from build123d import *

# Parameters (mm, degrees)
MAIN_DEPTH         = 5
SKETCH2_R          = 1.25
FIXHOLE1_DEPTH     = 51
SKETCH3_R          = 1.25
FIXHOLE2_DEPTH     = 51
WINDOWSLOT1_DEPTH  = 2
SKETCH6_R          = 1.25
CUT_EXTRUDE2_DEPTH = 3
LPATTERN1_COUNT    = 5
LPATTERN1_PITCH    = 10
SKETCH7_R          = 1.25
CUT_EXTRUDE3_DEPTH = 11
LPATTERN2_COUNT    = 4
LPATTERN2_PITCH    = 14.142


with BuildPart() as part:
    # Sketch1 → Main (new body, symmetric)
    with BuildSketch(Plane.XY):
        Polygon((-25, -25), (25, 25), (25, 15), (35, 15), (35, 10), (25, 10), (-10, -25), (-10, -35), (-15, -35), (-15, -25), align=None)
    extrude(amount=MAIN_DEPTH, both=True)

    # Sketch2 → FixHole1 (cut, through all)
    with BuildSketch(Plane(origin=(25, 0, 0), x_dir=(0, 0, -1), z_dir=(1, 0, 0))):
        with Locations((0, -30)):
            Circle(SKETCH2_R)
        with Locations((0, 20)):
            Circle(SKETCH2_R)
    extrude(amount=-FIXHOLE1_DEPTH, mode=Mode.SUBTRACT)

    # Sketch3 → FixHole2 (cut, through all)
    with BuildSketch(Plane(origin=(0, -25, 0), x_dir=(-1, 0, 0), z_dir=(0, -1, 0))):
        with Locations((20, 0)):
            Circle(SKETCH3_R)
        with Locations((-30, 0)):
            Circle(SKETCH3_R)
    extrude(amount=-FIXHOLE2_DEPTH, mode=Mode.SUBTRACT)

    # Sketch4 → WindowSlot1 (cut)
    with BuildSketch(Plane.XY.offset(5)):
        Polygon((25, 22.171572875), (-22.171572875, -25), (-18.636038969, -25), (25, 18.636038969), align=None)
    extrude(amount=-WINDOWSLOT1_DEPTH, mode=Mode.SUBTRACT)

    # Sketch6 → Cut-Extrude2 (cut)
    with BuildSketch(Plane(origin=(7.5, -7.5, 0), x_dir=(0, 0, 1), z_dir=(-0.707106781, 0.707106781, 0))):
        with Locations((0, 20)):
            Circle(SKETCH6_R)
    cut_extrude2 = extrude(amount=CUT_EXTRUDE2_DEPTH, mode=Mode.SUBTRACT)

    # LPattern1: Cut-Extrude2 ×5
    with Locations(*[Vector(-0.707106781, -0.707106781, 0) * (i * LPATTERN1_PITCH) for i in range(1, LPATTERN1_COUNT)]):
        add(cut_extrude2, mode=Mode.SUBTRACT)

    # Sketch7 → Cut-Extrude3 (cut, through all)
    with BuildSketch(Plane(origin=(0, 0, -5), x_dir=(-1, 0, 0), z_dir=(0, 0, -1))):
        with Locations((10, -20)):
            Circle(SKETCH7_R)
    cut_extrude3 = extrude(amount=-CUT_EXTRUDE3_DEPTH, mode=Mode.SUBTRACT)

    # LPattern2: Cut-Extrude3 ×4
    with Locations(*[Vector(0.707106781, 0.707106781, 0) * (i * LPATTERN2_PITCH) for i in range(1, LPATTERN2_COUNT)]):
        add(cut_extrude3, mode=Mode.SUBTRACT)


solid = part.part
CAD build for the part. Positions are in the model's coordinates, mm. A direction names the side the tool comes from. Give positions to 0.01 mm unless a question says otherwise; leave off trailing zeros. Write each loop counter-clockwise with the first axis right and the second up, starting at its lowest first coordinate (ties: lowest second). Pieces come first, ordered by that corner, then holes. Notation, with made-up numbers: (-10, -15.5) - (41, -15.5) arc R16 ccw to (41, 13.5) - close; hole circle Ø10 at (16, 26.5). An arc over 180 degrees is marked (long way). Answer as CSV lines item,"result".
Q1. Flat gauge pins, fed straight in: pin 1 Ø2 at (x, z) = (30, 0) entering from +Y; pin 2 Ø10 at (x, y) = (-6.5, 0) entering from -Z; pin 3 Ø2 at (x, z) = (15, -1) entering from -Y; pin 4 Ø2 at (x, z) = (10, 3.5) entering from -Y. Where does each tip first touch, or does it go through?
Result set:
pin 1,"through"
pin 2,"z = -5"
pin 3,"y = -1"
pin 4,"y = -6"
Q2. Pull direction X, two halves, no side cores. Call faces 4 (the face through (35, 13, 0)), 5 (the face through (-12, -35, 0)), 6 (the face through (0.26, -12.65, -0.16)): released by +X, released by -X, zero draft, split by the parting line, or undercut.
Result set:
face 4,"released by +X"
face 5,"zero draft"
face 6,"undercut"
Q3. Drill centre lines: line 1 (Z direction, x = 23, y = 20); line 2 (X direction, y = -9, z = 0.25); line 3 (Y direction, x = -17, z = 4.75). Where is each one in solid material? Low to high. Write a range as from..to.
Result set:
line 1,"-5..-1.25, 1.25..3"
line 2,"-9..-0.75, 0.75..6"
line 3,"-25..-23.36, -19.83..-17"
Q4. Band-saw the part on B-B (y = -30). Give the cut face in (x, z).
Result set:
outline,"(-15, -5) - (-10, -5) - (-10, -1.25) - (-15, -1.25) - close; (-15, 1.25) - (-10, 1.25) - (-10, 5) - (-15, 5) - close"
Q5. 3-axis set-ups, long thin cutter, end or side, ignore diameter. For faces 1 (the face through (1.744, -1.084, 4.014)), 2 (the face through (31, 15, 1)), 3 (the face through (-19, -25, -1)): which of +Z, -Z, +X, -X, +Y, -Y reach the whole face in a straight line?
Result set:
face 1,"+Z"
face 2,"+Z, -Z, +X, +Y"
face 3,"+Z, -Z, -X, -Y"
Q6. Band-saw the part on D-D (x = 24). Give the cut face in (y, z).
Result set:
outline,"(9, -5) - (24, -5) - (24, 5) - (21.17, 5) - (21.17, 3) - (17.64, 3) - (17.64, 5) - (9, 5) - close; hole circle Ø2.5 at (20, 0)"
Q7. Band-saw the part on A-A (x = 30). Give the cut face in (y, z).
Result set:
outline,"(10, -5) - (15, -5) - (15, -1.25) - (10, -1.25) - close; (10, 1.25) - (15, 1.25) - (15, 5) - (10, 5) - close"
Q8. Band-saw the part on C-C (z = -3). Give the cut face in (x, y), and give its area (3 significant figures).
Result set:
outline,"(-25, -25) - (-15, -25) - (-15, -35) - (-10, -35) - (-10, -25) - (25, 10) - (35, 10) - (35, 15) - (25, 15) - (25, 25) - close; hole circle Ø2.5 at (-10, -20); hole circle Ø2.5 at (0, -10); hole circle Ø2.5 at (10, 0); hole circle Ø2.5 at (20, 10)"
area,"718 mm²"
